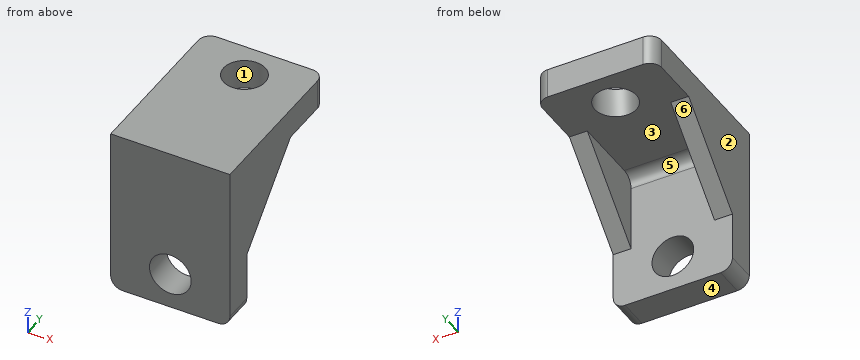
from build123d import *

# Parameters (mm, degrees)
BOSS_EXTRUDE3_DEPTH = 20
BOSS_EXTRUDE4_DEPTH = 3
BOSS_EXTRUDE5_DEPTH = 3
FILLET5_R           = 2
CUT_EXTRUDE1_REACH  = 43.388
SKETCH6_R           = 3.5
CUT_EXTRUDE2_REACH  = 43.388
SKETCH7_R           = 3.5


with BuildPart() as part:
    # Sketch3 → Boss-Extrude3 (new body)
    with BuildSketch(Plane(origin=(0, 0, 0), x_dir=(0, 0, -1), z_dir=(1, 0, 0))):
        Polygon((0, 0), (0, 28), (5, 28), (5, 5), (28, 5), (28, 0), align=None)
    extrude(amount=BOSS_EXTRUDE3_DEPTH)

    # Sketch4 → Boss-Extrude4 (add)
    with BuildSketch(Plane(origin=(20, 0, 0), x_dir=(0, 0, -1), z_dir=(1, 0, 0))):
        Polygon((5, 18), (5, 5), (18, 5), align=None)
    extrude(amount=-BOSS_EXTRUDE4_DEPTH)

    # Sketch5 → Boss-Extrude5 (add)
    with BuildSketch(Plane.ZY):
        Polygon((-5, 18), (-5, 5), (-18, 5), align=None)
    extrude(amount=-BOSS_EXTRUDE5_DEPTH)

    # Fillet5
    fillet5_edges = [part.edges().sort_by_distance(p)[0] for p in [
        (20, 28, -2.5),
        (10, 5, -5),
        (0, 28, -2.5),
        (0, 2.5, -28),
        (20, 2.5, -28),
    ]]
    fillet(fillet5_edges, radius=FILLET5_R)

    # Sketch6 → Cut-Extrude1 (cut, up to next)
    with BuildSketch(Plane(origin=(0, 0, -5), x_dir=(-1, 0, 0), z_dir=(0, 0, -1)), mode=Mode.PRIVATE) as cut_extrude1_sk1:
        with Locations(Location((-10, 22, 0), (0, 0, 90))):
            Circle(SKETCH6_R)
    cut_extrude1_tool1 = extrude(cut_extrude1_sk1.sketch, amount=-CUT_EXTRUDE1_REACH, mode=Mode.PRIVATE) & part.part
    add(cut_extrude1_tool1.solids().sort_by_distance((10, 22, -5))[0], mode=Mode.SUBTRACT)

    # Sketch7 → Cut-Extrude2 (cut, up to next)
    with BuildSketch(Plane(origin=(0, 5, 0), x_dir=(1, 0, 0), z_dir=(0, 1, 0)), mode=Mode.PRIVATE) as cut_extrude2_sk1:
        with Locations(Location((10, 22, 0), (0, 0, 270))):
            Circle(SKETCH7_R)
    cut_extrude2_tool1 = extrude(cut_extrude2_sk1.sketch, amount=-CUT_EXTRUDE2_REACH, mode=Mode.PRIVATE) & part.part
    add(cut_extrude2_tool1.solids().sort_by_distance((10, 5, -22))[0], mode=Mode.SUBTRACT)


solid = part.part
Work out the finished part from the listing and answer in its coordinate system (mm). Face numbers are marked on the shaded views. A direction names the side the tool comes from. Coordinates: 2 decimals unless noted, no trailing zeros. Write each loop counter-clockwise with the first axis right and the second up, starting at its lowest first coordinate (ties: lowest second). Pieces come first, ordered by that corner, then holes. Notation, with made-up numbers: M 87,54 L 91,54 A24 cw 91,92 Z; hole C -38.75,83 d5. An arc over 180 degrees is marked long. Answer as CSV lines item,"result". Start each with the question number.
Item 1: Consider L1, parallel to X at y = 7.5, z = -15; L2, parallel to X at y = 2.6, z = -22; L3, parallel to Y at x = 10.5, z = -14. Determine where each line is inside the solid, lowest interval first.
Item 2: Section B-B on y = 3.5 is taken. Write down the section's boundary in (x, z).
Item 3: Flat-ended cylindrical pins translate along their axes: P1, Ø3, axis at x = 12, z = -17, coming from the +Y side; P2, Ø6, axis at x = 7.5, y = 19.5, coming from the -Z side. Find the tip coordinate at first contact, or state that the pin passes through.
Item 4: Section A-A on x = 10 is taken. Write down the section's boundary in (y, z).
Item 5: A tool of negligible diameter and unlimited length cuts with its end or side. For the marked faces 5 and 6, from which of +Z, -Z, +X, -X, +Y, -Y can it reach the whole face along a straight path? Write none if from no direction.
Item 6: Section C-C on z = -22 is taken. Write down the section's boundary in (x, y).
Item 7: Section D-D on y = 15 is taken. Write down the section's boundary in (x, z), and give its area (3 significant figures).
Item 8: Determine the mould class of the marked faces 1, 2, 3 and 4 for opening direction X: released by +X, released by -X, zero draft, split by the parting line, or undercut.
Checks:
1,L1,"x = 0 to 3, 17 to 20"
1,L2,"x = 0 to 6.5, 13.5 to 20"
1,L3,"y = 0 to 5"
2,outline,"M 0,-26 A2 ccw 2,-28 L 18,-28 A2 ccw 20,-26 L 20,0 L 0,0 Z; hole C 10,-22 d7"
3,P1,"stops at y = 5"
3,P2,"stops at z = -5"
4,outline,"M 0,-28 L 5,-28 L 5,-25.5 L 0,-25.5 Z; M 0,-18.5 L 5,-18.5 L 5,-7 A2 cw 7,-5 L 18.5,-5 L 18.5,0 L 0,0 Z; M 25.5,-5 L 28,-5 L 28,0 L 25.5,0 Z"
5,face 5,"-Z, +Y"
5,face 6,"-Z, +X, -X, +Y"
6,outline,"M 0,0 L 6.5,0 L 6.5,5 L 0,5 Z; M 13.5,0 L 20,0 L 20,5 L 13.5,5 Z"
7,outline,"M 0,-8 L 3,-8 L 3,-5 L 17,-5 L 17,-8 L 20,-8 L 20,0 L 0,0 Z"
7,area,"118 mm²"
8,face 1,"undercut"
8,face 2,"released by -X"
8,face 3,"undercut"
8,face 4,"zero draft"
